Geometry: final body of the model. Coordinates: model frame, mm. A direction names the side the tool comes from. Give positions to 0.01 mm unless a question says otherwise; leave off trailing zeros. Write each loop counter-clockwise with the first axis right and the second up, starting at its lowest first coordinate (ties: lowest second). Pieces come first, ordered by that corner, then holes. Notation, with made-up numbers: M -4,39 L 30,39 A22 ccw 30,53 Z; hole C 73,-11 d2. An arc over 180 degrees is marked long. Use a Markdown table: item, result. Add a question column.
(1) Cut plane B-B (z = 0). Output: boundary loops of the cut face in (x, y) (3 decimals).
(2) Pin query (flat end, axial travel): pin 1 Ø1.5 at (x, y) = (-2.5, 3.5) entering from -Z; pin 2 Ø3 at (y, z) = (2, -8) entering from +X; pin 3 Ø4 at (x, y) = (-3.5, 11.5) entering from -Z. Return the tip coordinate at first contact, or that it passes through.
(3) Reachability of faces 1 (the cylindrical face through (3.82, 5.4, 1.2)), 2 (the flat face through (-5.8, 11, 7.3)) from +Z, -Z, +X, -X, +Y, -Y: full face, straight path, thin tool, end or side. Return the list, or none.
(4) Cut plane D-D (x = 8.5). Output: boundary loops of the cut face in (y, z).
(5) Material intervals for L1, parallel to Z at x = 0, y = 8.25 (3 decimals); L2, parallel to Y at x = 9.75, z = 2.5; L3, parallel to Z at x = 2, y = -0.75, sorted ascending.
(6) Draft query along Y for faces 3 (the cylindrical face through (-2.38, -0.99, -10.74)), 4 (the cylindrical face through (-1.99, 5.42, 8.95)), 5 (the flat face through (0, 13, 5)), 6 (the flat face through (0, -2, -5)). Return one class per face: released by +Y, released by -Y, zero draft, split by the parting line, or undercut.
(7) Cut plane C-C (y = -0.5). Output: boundary loops of the cut face in (x, z) (3 decimals), plus the area to 3 significant figures.
(8) Cut plane A-A (x = 0). Output: boundary loops of the cut face in (y, z) (3 decimals).
```python
from build123d import *

# Parameters (mm, degrees)
SKETCH_1_R          = 9.17
EXTRUDE_2_DEPTH     = 11
SKETCH_3_R          = 11
EXTRUDE_3_DEPTH     = 2
SKETCH_4_R          = 11
EXTRUDE_4_DEPTH     = 2
SKETCH_5_R          = 4.005
CUT_EXTRUDE_2_DEPTH = 16


with BuildPart() as part:
    # 草图1 → 凸台-拉伸2 (new body)
    with BuildSketch(Plane(origin=(0, 0, 0), x_dir=(1, 0, 0), z_dir=(0, 1, 0))):
        Circle(SKETCH_1_R)
    extrude(amount=EXTRUDE_2_DEPTH)

    # 草图3 → 凸台-拉伸3 (add)
    with BuildSketch(Plane(origin=(0, 11, 0), x_dir=(1, 0, 0), z_dir=(0, 1, 0))):
        Circle(SKETCH_3_R)
    extrude(amount=EXTRUDE_3_DEPTH)

    # 草图4 → 凸台-拉伸4 (add)
    with BuildSketch(Plane.XZ):
        Circle(SKETCH_4_R)
    extrude(amount=EXTRUDE_4_DEPTH)

    # 草图5 → 切除-拉伸2 (cut, through all)
    with BuildSketch(Plane.XZ.offset(2)):
        Circle(SKETCH_5_R)
    extrude(amount=-CUT_EXTRUDE_2_DEPTH, mode=Mode.SUBTRACT)


solid = part.part
```
Answer list:
| question | item | result |
|---|---|---|
| 1 | outline | M -11,-2 L -4.005,-2 L -4.005,13 L -11,13 L -11,11 L -9.17,11 L -9.17,0 L -11,0 Z; M 4.005,-2 L 11,-2 L 11,0 L 9.17,0 L 9.17,11 L 11,11 L 11,13 L 4.005,13 Z |
| 2 | pin 1 | z = -9 |
| 2 | pin 2 | x = 6.47 |
| 2 | pin 3 | z = -10.9 |
| 3 | face 1 | +Y, -Y |
| 3 | face 2 | none |
| 4 | outline | M -2,-6.98 L 0,-6.98 L 0,-3.44 L 11,-3.44 L 11,-6.98 L 13,-6.98 L 13,6.98 L 11,6.98 L 11,3.44 L 0,3.44 L 0,6.98 L -2,6.98 Z |
| 5 | L1 | -9.17 to -4.005, 4.005 to 9.17 |
| 5 | L2 | -2 to 0, 11 to 13 |
| 5 | L3 | -10.82 to -3.47, 3.47 to 10.82 |
| 6 | face 3 | zero draft |
| 6 | face 4 | undercut |
| 6 | face 5 | released by +Y |
| 6 | face 6 | released by -Y |
| 7 | outline | C 0,0 d22; hole C 0,0 d8.01 |
| 7 | area | 330 mm² |
| 8 | outline | M -2,-11 L 0,-11 L 0,-9.17 L 11,-9.17 L 11,-11 L 13,-11 L 13,-4.005 L -2,-4.005 Z; M -2,4.005 L 13,4.005 L 13,11 L 11,11 L 11,9.17 L 0,9.17 L 0,11 L -2,11 Z |
